Check sheet for the drawn part. Datum: minimum x, y, z corner. Units: mm. Round coordinates to 2 decimals unless told otherwise and drop trailing zeros. Order: outer loops, then holes, each group sorted by start corner. A loop starts at its lowest first (then second) coordinate and runs counter-clockwise, first axis right, second up. Notation, with made-up numbers: (59, 70) -> (116, 70) arc R27 ccw to (116, 95) -> close; hole circle Ø1 at (-8.75, 0). An arc over 180 degrees is marked (long way). Answer as a JSON object with one key per item and string values. Group by question number.
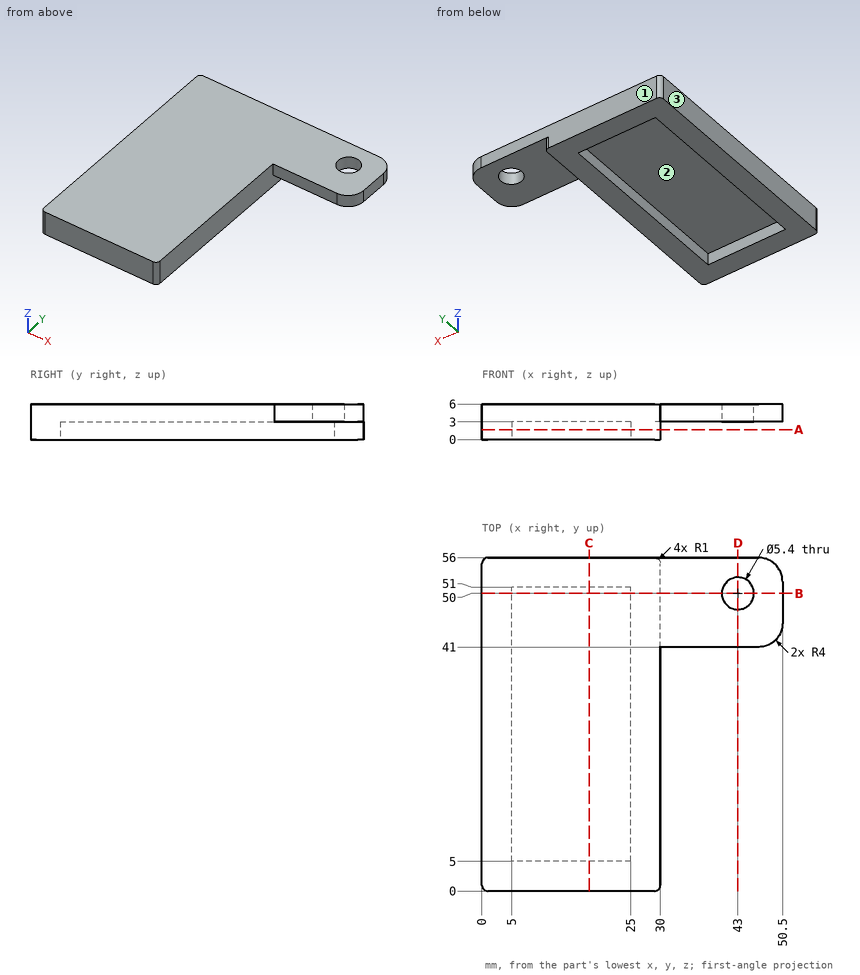
Item 1: Sectioned sample at A-A, the plane z = 1.7. Enter the section's corners in (x, y).
Item 2: Mould release check, pull along X, two halves, no side actions. Record for the marked faces 1, 2 and 3: pulls with the +X half, pulls with the -X half, needs draft (parallel to the pull), parting line crosses it, or undercut.
Item 3: Depth check by flat-ended pin: pin 1 Ø0.9 at (y, z) = (25.5, 1.5) entering from +X; pin 2 Ø7.5 at (x, y) = (42, 50) entering from -Z; pin 3 Ø3.5 at (x, z) = (36, 4) entering from -Y. Enter the tip coordinate at first touch or a pass-through.
Item 4: Sectioned sample at B-B, the plane y = 50. Enter the section's corners in (x, z).
Item 5: Sectioned sample at D-D, the plane x = 43. Enter the section's corners in (y, z), then the cut area to 3 significant figures.
Item 6: Thickness scan on L1, parallel to Y at x = 43, z = 5.1; L2, parallel to X at y = 39, z = 1.75; L3, parallel to Y at x = 11, z = 1.25. Record the ranges inside material, lowest first.
Item 7: Sectioned sample at C-C, the plane x = 18. Enter the section's corners in (y, z), then the cut area to 3 significant figures.
Result:
{
 "1": {"outline": "(0, 1) arc R1 ccw to (1, 0) -> (29, 0) arc R1 ccw to (30, 1) -> (30, 55) arc R1 ccw to (29, 56) -> (1, 56) arc R1 ccw to (0, 55) -> close; hole (5, 5) -> (25, 5) -> (25, 51) -> (5, 51) -> close"},
 "2": {"face 1": "needs draft", "face 2": "undercut", "face 3": "pulls with the -X half"},
 "3": {"pin 1": "stops at x = 30", "pin 2": "stops at z = 3", "pin 3": "stops at y = 41"},
 "4": {"outline": "(0, 0) -> (5, 0) -> (5, 3) -> (25, 3) -> (25, 0) -> (30, 0) -> (30, 3) -> (40.3, 3) -> (40.3, 6) -> (0, 6) -> close; (45.7, 3) -> (50.5, 3) -> (50.5, 6) -> (45.7, 6) -> close"},
 "5": {"outline": "(41, 3) -> (47.3, 3) -> (47.3, 6) -> (41, 6) -> close; (52.7, 3) -> (56, 3) -> (56, 6) -> (52.7, 6) -> close", "area": "28.8 mm2"},
 "6": {"L1": "y = 41 to 47.3, 52.7 to 56", "L2": "x = 0 to 5, 25 to 30", "L3": "y = 0 to 5, 51 to 56"},
 "7": {"outline": "(0, 0) -> (5, 0) -> (5, 3) -> (51, 3) -> (51, 0) -> (56, 0) -> (56, 6) -> (0, 6) -> close", "area": "198 mm2"}
}
